Could you check a few things on this model? Use its own coordinates, in mm. A direction names the side the tool comes from. Give positions to 0.01 mm unless a question says otherwise; leave off trailing zeros. Write each loop counter-clockwise with the first axis right and the second up, starting at its lowest first coordinate (ties: lowest second). Pieces come first, ordered by that corner, then holes. Notation, with made-up numbers: (69.25, 36.5) - (121.25, 36.5) arc R22 ccw to (121.25, 74.5) - close; hole circle Ø9 at (-23, 53.25). An arc over 180 degrees is marked (long way). Write item = value, one per line.
from build123d import *

# Parameters (mm, degrees)
F0_W     = 609.6
F0_H     = 304.8
F1_DEPTH = 12.7
F2_W     = 12.7
F2_H     = 304.8
F3_DEPTH = 304.8
F4_W     = 609.6
F4_H     = 317.5
F5_DEPTH = 12.7


with BuildPart() as f1:
    # F0 (on Front) → F1 (new body)
    with BuildSketch(Plane.XZ):
        with Locations((0, 152.4)):
            Rectangle(F0_W, F0_H)
    extrude(amount=F1_DEPTH)

    # F2 (on face) → F3 (join)
    with BuildSketch(Plane.XZ.offset(12.7)):
        with Locations((-158.75, 152.4)):
            Rectangle(F2_W, F2_H)
        with Locations((158.75, 152.4)):
            Rectangle(F2_W, F2_H)
    extrude(amount=F3_DEPTH)

    # F4 (on face) → F5 (join)
    with BuildSketch(Plane.XY.offset(304.8)):
        with Locations((0, -158.75)):
            Rectangle(F4_W, F4_H)
    extrude(amount=F5_DEPTH)


solid = f1.part
1. Which directions (+Z, -Z, +X, -X, +Y, -Y) give clear straight access to the entire face, cutting with the end or side of a thin tool? Please do faces 5 (the face through (234, -163, 304.8)), 6 (the face through (-236, -12.7, 155)), 7 (the face through (-2, -163, 304.8)).
Filled sheet:
face_5 = -Z, +X, -Y
face_6 = -Z, -X, -Y
face_7 = -Z, -Y
2. If we section it at C-C, the plane x = -118: Please give me the cut outline in (y, z).
Filled sheet:
outline = (-317.5, 304.8) - (-12.7, 304.8) - (-12.7, 0) - (0, 0) - (0, 317.5) - (-317.5, 317.5) - close
3. For pin 1 (8 mm diameter, centred on y = -67.5, z = 184, fed in from +X); pin 2 (5 mm diameter, centred on x = -118.5, z = 185, fed in from -Y); pin 3 (10 mm diameter, centred on y = -50, z = 279, fed in from -X), each with a flat end and sliding along its axis, tell me the tip position at first contact or that it passes through.
Filled sheet:
pin_1 = 165.1
pin_2 = -12.7
pin_3 = -165.1
4. I need wall thicknesses on line 1 (X direction, y = -283, z = 110); line 2 (Z direction, x = 12.5, y = -37); line 3 (Y direction, x = 97, z = 146.5). Which ranges of each line are inside material? Lowest first, please.
Filled sheet:
line_1 = -165.1 to -152.4, 152.4 to 165.1
line_2 = 304.8 to 317.5
line_3 = -12.7 to 0
5. Thinking about a two-plate mould opening in X: for faces 1 (the face through (-165.1, -163, 150)), 2 (the face through (-1, -317.5, 311)), 3 (the face through (-2, -12.7, 155)), 4 (the face through (304.8, -7, 229)), which applies, pulls with the +X half, pulls with the -X half, needs draft (parallel to the pull), parting line crosses it, or undercut?
Filled sheet:
face_1 = pulls with the -X half
face_2 = needs draft
face_3 = undercut
face_4 = pulls with the +X half
6. If we section it at A-A, the plane y = -63: Please give me the cut outline in (x, z), and give its area (3 significant figures).
Filled sheet:
outline = (-304.8, 304.8) - (-165.1, 304.8) - (-165.1, 0) - (-152.4, 0) - (-152.4, 304.8) - (152.4, 304.8) - (152.4, 0) - (165.1, 0) - (165.1, 304.8) - (304.8, 304.8) - (304.8, 317.5) - (-304.8, 317.5) - close
area = 15,500 mm2
7. If we section it at B-B, the plane z = 60.5: Please give me the cut outline in (x, y).
Filled sheet:
outline = (-304.8, -12.7) - (-165.1, -12.7) - (-165.1, -317.5) - (-152.4, -317.5) - (-152.4, -12.7) - (152.4, -12.7) - (152.4, -317.5) - (165.1, -317.5) - (165.1, -12.7) - (304.8, -12.7) - (304.8, 0) - (-304.8, 0) - close
